Design review of the part built by this model. Coordinates are the model's own, in mm. Face numbers are marked on the shaded views. A direction names the side the tool comes from. Coordinates: 2 decimals unless noted, no trailing zeros. Loops run counter-clockwise (first coordinate to the right, second up) from the corner with the lowest first, then second, coordinate; pieces in that order, holes last. Notation, with made-up numbers: M 35.5,-38 L 44.5,-38 A27 ccw 44.5,-14 Z; hole C 26,64.25 d9. An arc over 180 degrees is marked long. One line per item, written item: value.
```python
from build123d import *

# Parameters (mm, degrees)
SKETCH1_W           = 15
SKETCH1_H           = 15
BOSS_EXTRUDE1_DEPTH = 15
SKETCH2_W           = 10
SKETCH2_H           = 10
BOSS_EXTRUDE2_DEPTH = 5
SKETCH3_R           = 2.5
CUT_EXTRUDE1_DEPTH  = 25.852419528
FILLET1_R           = 2


with BuildPart() as part:
    # Sketch1 → Boss-Extrude1 (new body)
    with BuildSketch(Plane(origin=(0, 0, 0), x_dir=(1, 0, 0), z_dir=(0, 1, 0))):
        with Locations((5.447693091, -2.5)):
            Rectangle(SKETCH1_W, SKETCH1_H)
    extrude(amount=BOSS_EXTRUDE1_DEPTH)

    # Sketch2 → Boss-Extrude2 (add)
    with BuildSketch(Plane.XZ):
        with Locations((5.447693091, 2.5)):
            Rectangle(SKETCH2_W, SKETCH2_H)
    extrude(amount=BOSS_EXTRUDE2_DEPTH)

    # Sketch3 → Cut-Extrude1 (cut, through all)
    with BuildSketch(Plane.XY.offset(10)):
        with Locations((5.447693091, 7.5)):
            Circle(SKETCH3_R)
    extrude(amount=-CUT_EXTRUDE1_DEPTH, mode=Mode.SUBTRACT)

    # Fillet1
    fillet1_edges = [part.edges().sort_by_distance(p)[0] for p in [
        (-2.052306909, 15, 2.5),
        (5.447693091, 15, 10),
        (12.947693091, 15, 2.5),
        (5.447693091, 0, 10),
        (-2.052306909, 0, 2.5),
        (5.447693091, 0, -5),
        (12.947693091, 0, 2.5),
        (12.947693091, 7.5, 10),
        (-2.052306909, 7.5, 10),
        (-2.052306909, 7.5, -5),
        (12.947693091, 7.5, -5),
        (5.447693091, 15, -5),
    ]]
    fillet(fillet1_edges, radius=FILLET1_R)


solid = part.part
```
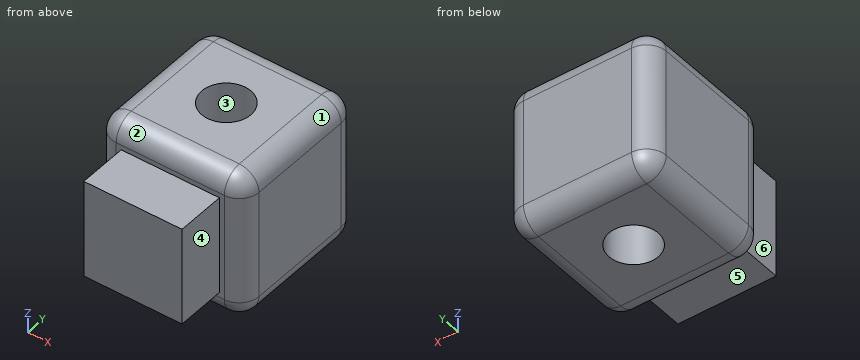
(1) Mouldability with a two-part tool opening along Y and no side actions: class the marked faces 1, 2 and 3 as released by +Y, released by -Y, zero draft, split by the parting line, or undercut.
Reply:
face 1: zero draft
face 2: released by -Y
face 3: undercut
(2) Tool access review of the marked faces 4, 5 and 6: name each direction out of +Z, -Z, +X, -X, +Y, -Y from which nothing blocks a thin tool from reaching the whole face with its end or side.
Reply:
face 4: +Z, -Z, +X, -Y
face 5: -Z, +X, -X, -Y
face 6: +Z, -Z, -X, -Y
(3) To check wall thickness, follow line 1 along Y through (x, z) = (7.75, 8.25); line 2 along Y through (x, z) = (7.5, 5.5); line 3 along X through (y, z) = (7.75, 3). State the ranges of each line that lie inside material, in increasing order. Write a range as [from, to].
Reply:
line 1: y = [0.02, 6.53], [8.47, 14.98]
line 2: y = [-5, 6.07], [8.93, 15]
line 3: x = [-2.05, 2.96], [7.94, 12.95]
(4) We need section A-A on y = 7.5. State the section outline as (x, z) points.
Reply:
outline: M -2.05,-3 A2 ccw -0.05,-5 L 2.95,-5 L 2.95,10 L -0.05,10 A2 ccw -2.05,8 Z; M 7.95,-5 L 10.95,-5 A2 ccw 12.95,-3 L 12.95,8 A2 ccw 10.95,10 L 7.95,10 Z
(5) Insertion check: pin 1 (4 mm diameter, centred on x = 3.5, y = -3.5, fed in from +Z); pin 2 (3 mm diameter, centred on x = 5.45, y = 7.5, fed in from +Z); pin 3 (2.5 mm diameter, centred on y = -3, z = 3, fed in from -X); pin 4 (4 mm diameter, centred on x = 7, y = -3, fed in from -Z). Each pin has a flat end and moves straight along its axis. Give the tip position at first contact, or say it passes through.
Reply:
pin 1: stops at z = 7.5
pin 2: passes through
pin 3: stops at x = 0.45
pin 4: stops at z = -2.5
(6) We need section D-D on x = 7. State the section outline as (y, z) points.
Reply:
outline: M -5,-2.5 L 0,-2.5 L 0,-3 A2 ccw 2,-5 L 5.54,-5 L 5.54,10 L 2,10 A2 ccw 0,8 L 0,7.5 L -5,7.5 Z; M 9.46,-5 L 13,-5 A2 ccw 15,-3 L 15,8 A2 ccw 13,10 L 9.46,10 Z
(7) We need section B-B on z = 3.75. State the section outline as (x, y) points.
Reply:
outline: M -2.05,2 A2 ccw -0.05,0 L 0.45,0 L 0.45,-5 L 10.45,-5 L 10.45,0 L 10.95,0 A2 ccw 12.95,2 L 12.95,13 A2 ccw 10.95,15 L -0.05,15 A2 ccw -2.05,13 Z; hole C 5.45,7.5 d5
(8) We need section C-C on x = 8.75. State the section outline as (y, z) points, then the cut area to 3 significant figures.
Reply:
outline: M -5,-2.5 L 0,-2.5 L 0,-3 A2 ccw 2,-5 L 13,-5 A2 ccw 15,-3 L 15,8 A2 ccw 13,10 L 2,10 A2 ccw 0,8 L 0,7.5 L -5,7.5 Z
area: 272 mm2
